Autodesk Inventor part; units mm, degrees
ref_plane "YZ Plane" through (0, 0, 0) normal (1, 0, 0) x (0, 1, 0)
ref_plane "XZ Plane" through (0, 0, 0) normal (0, 1, 0) x (-1, 0, 0)
ref_plane "XY Plane" through (0, 0, 0) normal (0, 0, 1) x (1, 0, 0)
sketch "Sketch1" plane through (0, 0, 0) normal (0, 0, 1) x (1, 0, 0)
  line L0 (-254, 0) -> (254, 0)
  line L1 (-156.845, 1347.6224) -> (156.845, 1347.6224)
  line L2 (-156.845, 1347.6224) -> (-254, 0)
  line L3 (254, 0) -> (156.845, 1347.6224)
  point P0 (0, 0)
  point P1 (0, 0)
  point P2 (0, 1347.6224)
  dimension "d0" = 508
  dimension "d1" = 313.69
  dimension "d2" = 1347.6224
extrude "Plate1" add sketch "Sketch1" along normal blind 3.175
sketch "Sketch3" plane through (254, -3.1268, 6.9013) normal (0, -0.9848078, 0.1736482) x (1, 0, 0)
  line L0 (-508, 0) -> (0, 0)
  line L1 (0, 0) -> (0, 17.8324)
  line L2 (0, 17.8324) -> (-508, 17.8324)
  line L3 (-508, 17.8324) -> (-508, 0)
edge flange "Flange2" height 25.4 angle 100 thickness 3.175 bend radius 3.175 thickness toward (0, -0.9848078, 0.1736482) relief tear relief width 3.175 relief depth 1.5875 edges at (0, 0, 3.175) wall of the first edge with corners at (-254, -3.1268, 6.9013) (254, -3.1268, 6.9013) (254, -0.0302, 24.4628) (-254, -0.0302, 24.4628)
bend "Bend2"
corner "Corner2"
sketch "Sketch4" plane through (-254, -0.0302, 24.4628) normal (0, 0.9848078, -0.1736482) x (1, 0, 0)
  line L0 (508, 17.8324) -> (0, 17.8324)
  line L1 (508, 17.8324) -> (487.7938, 0)
  line L2 (0, 0) -> (508, 0)
  line L3 (487.7938, 0) -> (508, 0)
  line L4 (508, 0) -> (508, 17.8324)
  line L5 (508, 0) -> (508, 17.8324)
  line L6 (508, 17.8324) -> (487.7938, 0)
  point P0 (254, 24.0859)
extrude "Cut1" cut sketch "Sketch4" against normal blind 3.175
sketch "Sketch5" plane through (-254, -3.1268, 6.9013) normal (0, 0.9848078, -0.1736482) x (1, 0, 0)
  line L0 (0, -17.8324) -> (0, 0)
  line L1 (0, 0) -> (20.2032, -17.8324)
  line L2 (0, -17.8324) -> (487.7938, -17.8324)
  point P0 (254, 6.2535)
extrude "Cut2" cut sketch "Sketch5" against normal blind 3.175
equation "\"d24\" = Thickness"
equation "\"d26\" = Thickness"
equation "\"d14\" = BendReliefWidth"
equation "\"d15\" = BendReliefDepth"
equation "\"d16\" = MinimumRemnant"
equation "\"d17\" = BendRadius"
equation "\"d20\" = BendRadius"
equation "\"d21\" = CornerReliefSize"
equation "\"d22\" = GapSize"
equation "\"d23\" = JacobiRadiusSize"
equation "\"BendRadius\" = Thickness"
equation "\"BendReliefWidth\" = Thickness"
equation "\"BendReliefDepth\" = 0.5 * Thickness"
equation "\"CornerReliefSize\" = 4 * Thickness"
equation "\"MinimumRemnant\" = 2 * Thickness"
equation "\"TransitionRadius\" = BendRadius"
equation "\"JacobiRadiusSize\" = BendRadius"
equation "\"GapSize\" = Thickness"
equation "\"d3\" = BendRadius"
properties part number "robot side"
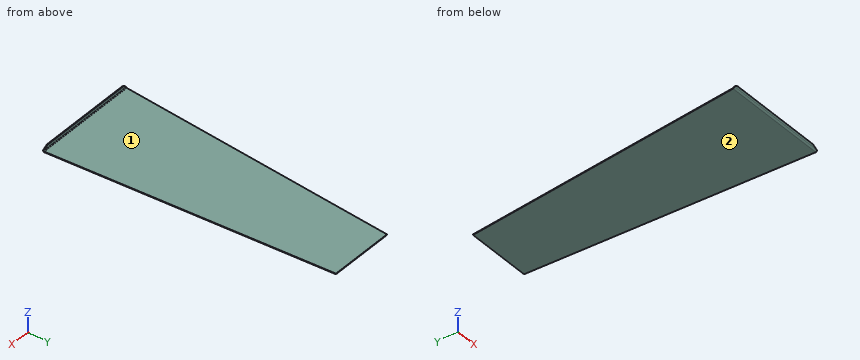
Could you check a few things on this model? Use its own coordinates, in mm. Face numbers are marked on the shaded views. A direction names the side the tool comes from. Give positions to 0.01 mm unless a question says otherwise; leave off trailing zeros. Order: outer loops, then holes, each group sorted by start corner. A loop starts at its lowest first (then second) coordinate and runs counter-clockwise, first axis right, second up.
Item 1: If we section it at B-B, the plane z = 20.5: Write out the boundary of the cut face in (x, y), plus the area to 3 significant figures.
Item 2: If we section it at A-A, the plane x = -24.5: Write out the boundary of the cut face in (y, z) (3 decimals).
Item 3: If we section it at C-C, the plane y = 1123: Write out the boundary of the cut face in (x, z) (3 decimals).
Item 4: I need wall thicknesses on line 1 (Z direction, x = 232.5, y = 234) (3 decimals); line 2 (Y direction, x = 40, z = 5); line 3 (Y direction, x = -81, z = 11.75). Which ranges of each line are inside material? Lowest first, please.
Item 5: I'm going to push flat-ended pins straight in: pin 1 (5 mm diameter, centred on x = -115.5, z = 20, fed in from -Y); pin 2 (5 mm diameter, centred on x = -153.5, z = 14.5, fed in from -Y); pin 3 (4 mm diameter, centred on x = 36.5, z = 12, fed in from -Y). Where does each tip first touch, or does it pass through?
Item 6: For the marked faces 1 and 2, which set-ups out of +Z, -Z, +X, -X, +Y, -Y let a thin tool reach every point of the face, with its end or its side?
Values:
1. outline: (-238.99, -3.95) - (238.99, -3.95) - (238.35, -0.73) - (-238.36, -0.73) - close
1. area: 1,540 mm2
2. outline: (-6.254, 7.453) arc R6.35 ccw to (0, 0) - (1347.622, 0) - (1347.622, 3.175) - (0, 3.175) arc R3.175 cw to (-3.127, 6.901) - (-0.03, 24.463) - (-3.157, 25.014) - close
3. outline: (-173.039, 0) - (173.039, 0) - (173.039, 3.175) - (-173.039, 3.175) - close
4. line 1: z = 0 to 3.175
4. line 2: y = -6.2 to -2.87
4. line 3: y = -5.5 to -2.27
5. pin 1: stops at y = -4.48
5. pin 2: stops at y = -5.45
5. pin 3: stops at y = -5.8
6. face 1: +Z, +X, -X, +Y
6. face 2: -Z, +X, -X, +Y, -Y
